Check sheet for the modelled part. Datum: model origin and axes. Units: mm. Face numbers are marked on the shaded views. A direction names the side the tool comes from. Round coordinates to 2 decimals unless told otherwise and drop trailing zeros. Loops run counter-clockwise (first coordinate to the right, second up) from the corner with the lowest first, then second, coordinate; pieces in that order, holes last. Notation, with made-up numbers: M -9,65.25 L 21,65.25 A29 cw 21,100.25 Z; hole C 13.25,50.25 d10. An arc over 180 degrees is marked long. One line per question, with ' | ' between items. Start each with the question number.
(1) Section check D-D (x = -3.25). Count the separate pieces of the cut face and the enclosed holes in it, and give its area (3 significant figures).
(2) Go/stop test with flat-tipped pins: P1, Ø1.8, axis at x = -4, z = 22.5, coming from the +Y side; P2, Ø1.5, axis at x = -3.5, z = 15.5, coming from the +Y side; P3, Ø2.5, axis at y = 0, z = 22.5, coming from the +X side. Record where each tip stops, or that it passes through.
(3) Tool access check on the marked faces 1, 2, 3 and 4. Record the directions out of +Z, -Z, +X, -X, +Y, -Y that give a thin tool (end or side, any length) a straight path to the whole face; none if there is none.
(4) Section check C-C (z = 19.25). Record the boundary of the cut face in (x, y).
(5) Section check A-A (x = 1). Record the boundary of the cut face in (y, z).
(6) Thickness scan on probe 1 along Z at (x, y) = (1.05, 0); probe 2 along Z at (x, y) = (0.5, 3.25); probe 3 along Z at (x, y) = (-0.2, 0). Record the ranges inside material, lowest first. Write a range as [from, to].
(7) Draft check along Z on the marked faces 5, 6 and 7. Enter one of: +Z half, -Z half, draft (parallel to the pull), parting line (faces both ways), or undercut.
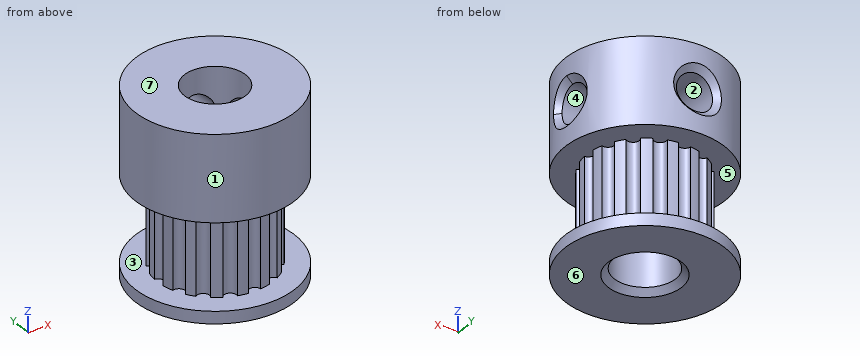
```python
from build123d import *

# Parameters (mm, degrees)
SKETCH068_R            = 0.5
PAD053_DEPTH           = 7
SKETCH067_R            = 1.5
PAD052_DEPTH           = 8
SKETCH066_R            = 1.5
PAD051_DEPTH           = 8
SKETCH065_R            = 2.5
POCKET001_DEPTH        = 15
CHAMFER002_SIZE        = 0.5
CHAMFER003_SIZE        = 0.5
CUT005_PLACEMENT_ANGLE = 180


with BuildPart() as pad053:
    # Sketch068 → Pad053 (new body)
    with BuildSketch(Plane.XY.offset(14)):
        with Locations((0, 4.7)):
            Circle(SKETCH068_R)
        with Locations((0, -4.7)):
            Circle(SKETCH068_R)
        with Locations((4.7, 0)):
            Circle(SKETCH068_R)
        with Locations((-4.7, 0)):
            Circle(SKETCH068_R)
        with Locations((-3.323402, 3.323402)):
            Circle(SKETCH068_R)
        with Locations((3.323402, 3.323402)):
            Circle(SKETCH068_R)
        with Locations((-3.323402, -3.323402)):
            Circle(SKETCH068_R)
        with Locations((3.323402, -3.323402)):
            Circle(SKETCH068_R)
        with Locations((-1.798612, 4.342234)):
            Circle(SKETCH068_R)
        with Locations((1.798612, 4.342234)):
            Circle(SKETCH068_R)
        with Locations((4.342234, 1.798612)):
            Circle(SKETCH068_R)
        with Locations((4.342234, -1.798612)):
            Circle(SKETCH068_R)
        with Locations((1.798612, -4.342234)):
            Circle(SKETCH068_R)
        with Locations((-1.798612, -4.342234)):
            Circle(SKETCH068_R)
        with Locations((-4.342234, -1.798612)):
            Circle(SKETCH068_R)
        with Locations((-4.314713, 1.863666)):
            Circle(SKETCH068_R)
    extrude(amount=-PAD053_DEPTH)


with BuildPart() as pad052:
    # Sketch067 → Pad052 (new body)
    with BuildSketch(Plane(origin=(7, 0, 3.5), x_dir=(0, 1, 0), z_dir=(1, 0, 0))):
        Circle(SKETCH067_R)
    extrude(amount=-PAD052_DEPTH)


with BuildPart() as pad051:
    # Sketch066 → Pad051 (new body)
    with BuildSketch(Plane(origin=(0, -7, 3.5), x_dir=(1, 0, 0), z_dir=(0, -1, 0))):
        Circle(SKETCH066_R)
    extrude(amount=-PAD051_DEPTH)


with BuildPart() as gt1_pulley001:
    # Sketch064 → Revolution004 (revolve)
    with BuildSketch(Plane.XZ):
        Polygon((0, 0), (6.5, 0), (6.5, 7), (4.7, 7), (4.7, 14), (6.5, 14), (6.5, 15), (0, 15), align=None)
    revolve(axis=Axis((0, 0, 0), (0, 0, 1)))

    # Sketch065 (on Face7 of Revolution004) → Pocket001 (cut)
    with BuildSketch(Plane(origin=(0, 0, 15), x_dir=(-1, 0, 0), z_dir=(0, 0, 1))):
        Circle(SKETCH065_R)
    extrude(amount=-POCKET001_DEPTH, mode=Mode.SUBTRACT)

    # Cut003: cut Pad051
    add(pad051.part, mode=Mode.SUBTRACT)

    # Cut004: cut Pad052
    add(pad052.part, mode=Mode.SUBTRACT)

    # Chamfer002
    chamfer002_edges = [gt1_pulley001.edges().sort_by_distance(p)[0] for p in [
        (-4e-06, -6.499997, 4.999986),
        (-4e-06, -6.499997, 2.000014),
        (6.412872, 1.060693, 4.560627),
        (6.412872, 1.060693, 2.439373),
        (6.412872, -1.060693, 2.439373),
        (6.412872, -1.060693, 4.560627),
    ]]
    chamfer(chamfer002_edges, length=CHAMFER002_SIZE)

    # Chamfer003
    chamfer003_edges = [gt1_pulley001.edges().sort_by_distance(p)[0] for p in [
        (2.5, 0, 15),
    ]]
    chamfer(chamfer003_edges, length=CHAMFER003_SIZE)

    # Cut005: cut Pad053
    add(pad053.part, mode=Mode.SUBTRACT)


with BuildPart() as gt1_pulley001_1:
    # Cut005 placement: moved
    add(gt1_pulley001.part.moved(Location((-4, 0, 26))).rotate(Axis((-4, 0, 26), (1, 0, 0)), CUT005_PLACEMENT_ANGLE))


solid = gt1_pulley001_1.part
```
The answers:
1) separate pieces: 3 | enclosed holes: 0 | area: 85.6 mm²
2) P1: y = -2.33 | P2: y = 4.67 | P3: x = -6.17
3) face 1: +Z, -Z | face 2: +Y | face 3: none | face 4: +X
4) outline: C -4,0 d13; hole C -4,0 d5
5) outline: M -4.15,11 L 4.15,11 L 4.15,12 L -4.15,12 Z; M -4.15,19 L 4.15,19 L 4.15,26 L -4.15,26 Z; hole C 0,22.5 d3
6) probe 1: [11, 12], [19, 21], [24, 26] | probe 2: [11, 12], [19, 26] | probe 3: [11, 21], [24, 26]
7) face 5: undercut | face 6: -Z half | face 7: +Z half
